```python
from build123d import *

# Parameters (mm, degrees)
BOSS_EXTRUDE1_DEPTH = 15.6
BOSS_EXTRUDE2_DEPTH = 6.75
BOSS_EXTRUDE3_DEPTH = 4
BOSS_EXTRUDE4_DEPTH = 3
SKETCH5_R           = 1.65
CUT_EXTRUDE1_DEPTH  = 8
SKETCH6_R           = 1.65
CUT_EXTRUDE2_DEPTH  = 27.35
CUT_EXTRUDE3_START  = -3
CUT_EXTRUDE3_DEPTH  = 2.6
CUT_EXTRUDE4_DEPTH  = 20
SKETCH9_W           = 15.8100889
SKETCH9_H           = 107.753083684
SKETCH9_W_2         = 8.2399111
SKETCH9_H_2         = 107.633309651
CUT_EXTRUDE5_DEPTH  = 10
SKETCH10_R          = 0.625
CUT_EXTRUDE6_DEPTH  = 30


with BuildPart() as part:
    # Sketch1 → Boss-Extrude1 (new body)
    with BuildSketch(Plane.XY):
        Polygon((-11.65, 6.6), (11.35, 6.6), (11.35, -6.2), (23.85, -6.2), (23.85, 8.35), (-24.15, 8.35), (-24.15, -6.2), (-11.65, -6.2), align=None)
    extrude(amount=-BOSS_EXTRUDE1_DEPTH)

    # Sketch2 → Boss-Extrude2 (add)
    with BuildSketch(Plane(origin=(0, 0, -15.6), x_dir=(-1, 0, 0), z_dir=(0, 0, -1))):
        Polygon((-16.2399111, -6.2), (-23.85, -6.2), (-23.85, 8.35), (24.2, 8.35), (24.2, -6.2), (16.0600889, -6.2), (16.0600889, 6.6), (-16.2399111, 6.6), align=None)
    extrude(amount=BOSS_EXTRUDE2_DEPTH)

    # Sketch3 → Boss-Extrude3 (add)
    with BuildSketch(Plane.XY):
        with BuildLine():
            Line((-24.15, 8.35), (23.85, 8.35))
            Line((23.85, 8.35), (23.85, 1.000334142))
            Line((23.85, 1.000334142), (23.85, -108.560334142))
            ThreePointArc((23.85, -108.560334142), (0.155860803, -114.961112509), (-24.15, -111.554159822))
            Line((-24.15, -111.554159822), (-24.15, 3.741161814))
            Line((-24.15, 3.741161814), (-24.15, 8.35))
        make_face()
    extrude(amount=BOSS_EXTRUDE3_DEPTH)

    # Sketch4 → Boss-Extrude4 (add)
    with BuildSketch(Plane(origin=(0, 0, 0), x_dir=(-1, 0, 0), z_dir=(0, 0, -1))):
        with BuildLine():
            ThreePointArc((10.093422233, -114.741481463), (13.037755905, -114.358456249), (15.9600889, -113.833309651))
            Line((15.9600889, -113.833309651), (15.9600889, -35.2))
            Line((15.9600889, -35.2), (10.093422233, -35.2))
            Line((10.093422233, -35.2), (10.093422233, -114.741481463))
        make_face()
        with BuildLine():
            ThreePointArc((1.026755567, -115.023412344), (3.960432973, -115.079264216), (6.893422233, -114.994667814))
            Line((6.893422233, -114.994667814), (6.893422233, -35.2))
            Line((6.893422233, -35.2), (1.026755567, -35.2))
            Line((1.026755567, -35.2), (1.026755567, -115.023412344))
        make_face()
        with BuildLine():
            ThreePointArc((-8.0399111, -113.953083684), (-5.116842896, -114.448405849), (-2.173244433, -114.801817592))
            Line((-2.173244433, -114.801817592), (-2.173244433, -35.2))
            Line((-2.173244433, -35.2), (-8.0399111, -35.2))
            Line((-8.0399111, -35.2), (-8.0399111, -113.953083684))
        make_face()
    extrude(amount=BOSS_EXTRUDE4_DEPTH)

    # Sketch5 → Cut-Extrude1 (cut, through all)
    with BuildSketch(Plane(origin=(0, 0, -3), x_dir=(-1, 0, 0), z_dir=(0, 0, -1))):
        with Locations((3.9600889, -46.2)):
            Circle(SKETCH5_R)
        with Locations((12.4600889, -46.2)):
            Circle(SKETCH5_R)
        with Locations((-4.5399111, -46.2)):
            Circle(SKETCH5_R)
        with Locations((12.4600889, -105.2)):
            Circle(SKETCH5_R)
        with Locations((-4.5399111, -105.2)):
            Circle(SKETCH5_R)
    extrude(amount=-CUT_EXTRUDE1_DEPTH, mode=Mode.SUBTRACT)

    # Sketch6 → Cut-Extrude2 (cut, through all)
    with BuildSketch(Plane(origin=(0, 0, -22.35), x_dir=(-1, 0, 0), z_dir=(0, 0, -1))):
        with Locations((-20.1399111, -2.18)):
            Circle(SKETCH6_R)
        with Locations((-20.1399111, 3.82)):
            Circle(SKETCH6_R)
        with Locations((19.9600889, -2.18)):
            Circle(SKETCH6_R)
        with Locations((19.9600889, 3.82)):
            Circle(SKETCH6_R)
    extrude(amount=-CUT_EXTRUDE2_DEPTH, mode=Mode.SUBTRACT)

    # Sketch7 → Cut-Extrude3 (cut)
    with BuildSketch(Plane(origin=(0, 0, -22.35), x_dir=(-1, 0, 0), z_dir=(0, 0, -1)).offset(CUT_EXTRUDE3_START)):
        Polygon((18.314640633, 0.67), (16.669192365, -2.18), (18.314640633, -5.03), (21.605537167, -5.03), (23.250985434, -2.18), (21.605537167, 0.67), align=None)
        Polygon((21.605537167, 6.67), (18.314640633, 6.67), (16.669192365, 3.82), (18.314640633, 0.97), (21.605537167, 0.97), (23.250985434, 3.82), align=None)
        Polygon((-21.785359367, 6.67), (-23.430807635, 3.82), (-21.785359367, 0.97), (-18.494462833, 0.97), (-16.849014566, 3.82), (-18.494462833, 6.67), align=None)
        Polygon((-21.785359367, 0.67), (-23.430807635, -2.18), (-21.785359367, -5.03), (-18.494462833, -5.03), (-16.849014566, -2.18), (-18.494462833, 0.67), align=None)
    extrude(amount=-CUT_EXTRUDE3_DEPTH, mode=Mode.SUBTRACT)

    # Sketch8 → Cut-Extrude4 (cut)
    with BuildSketch(Plane.ZY.offset(-11.35)):
        Polygon((0, 6.6), (-4.810139763, 6.6), (-8, 1.075), (-4.810139763, -4.45), (0, -4.45), align=None)
    extrude(amount=-CUT_EXTRUDE4_DEPTH, mode=Mode.SUBTRACT)

    # Sketch9 → Cut-Extrude5 (cut)
    with BuildSketch(Plane(origin=(0, 0, 0), x_dir=(-1, 0, 0), z_dir=(0, 0, -1))):
        with Locations((-15.94495555, -60.076541842)):
            Rectangle(SKETCH9_W, SKETCH9_H)
        with Locations((20.08004445, -60.016654826)):
            Rectangle(SKETCH9_W_2, SKETCH9_H_2)
    extrude(amount=-CUT_EXTRUDE5_DEPTH, mode=Mode.SUBTRACT)

    # Sketch10 → Cut-Extrude6 (cut)
    with BuildSketch(Plane(origin=(0, 0, -15.6), x_dir=(-1, 0, 0), z_dir=(0, 0, -1))):
        with Locations((13.8100889, 0.32)):
            Circle(SKETCH10_R)
        with Locations((-13.9899111, 0.32)):
            Circle(SKETCH10_R)
    extrude(amount=-CUT_EXTRUDE6_DEPTH, mode=Mode.SUBTRACT)


solid = part.part
```
Geometry: final body of the model. Coordinates: model frame, mm. A direction names the side the tool comes from. Coordinates: 2 decimals unless noted, no trailing zeros. Order: outer loops, then holes, each group sorted by start corner. A loop starts at its lowest first (then second) coordinate and runs counter-clockwise, first axis right, second up.
Item 1: Section query C-C (y = -46.2). Output: boundary loops of the cut face in (x, z).
Answer:
outline: (-15.96, -3) - (-14.11, -3) - (-14.11, 4) - (-15.96, 4) - close; (-10.81, -3) - (-10.09, -3) - (-10.09, 0) - (-6.89, 0) - (-6.89, -3) - (-5.61, -3) - (-5.61, 4) - (-10.81, 4) - close; (-2.31, -3) - (-1.03, -3) - (-1.03, 0) - (2.17, 0) - (2.17, -3) - (2.89, -3) - (2.89, 4) - (-2.31, 4) - close; (6.19, -3) - (8.04, -3) - (8.04, 4) - (6.19, 4) - close
Item 2: Contact query for flat-ended pins moving along their axis: P1, Ø3.5, axis at y = -58, z = -1, coming from the -X side; P2, Ø2, axis at x = 20, z = -17.5, coming from the -Y side; P3, Ø1, axis at x = -8.5, y = -88, coming from the -Z side. Output: stop coordinate, or through.
Answer:
P1: stops at x = -15.96
P2: stops at y = -6.2
P3: stops at z = 0
Item 3: Section query A-A (y = -105.2). Output: boundary loops of the cut face in (x, z), then the cut area to 3 significant figures.
Answer:
outline: (-15.96, -3) - (-14.11, -3) - (-14.11, 4) - (-15.96, 4) - close; (-10.81, -3) - (-10.09, -3) - (-10.09, 0) - (-6.89, 0) - (-6.89, -3) - (-1.03, -3) - (-1.03, 0) - (2.17, 0) - (2.17, -3) - (2.89, -3) - (2.89, 4) - (-10.81, 4) - close; (6.19, -3) - (8.04, -3) - (8.04, 4) - (6.19, 4) - close
area: 103 mm2
Item 4: Section query D-D (y = -75). Output: boundary loops of the cut face in (x, z), then the cut area to 3 significant figures.
Answer:
outline: (-15.96, -3) - (-10.09, -3) - (-10.09, 0) - (-6.89, 0) - (-6.89, -3) - (-1.03, -3) - (-1.03, 0) - (2.17, 0) - (2.17, -3) - (8.04, -3) - (8.04, 4) - (-15.96, 4) - close
area: 149 mm2
Item 5: Access query for faces 4 (the face through (-5, -53, 4)), 5 (the face through (20.5, -3.79, -11.03)), 6 (the face through (18.7, -0.9, -19.35)), 7 (the face through (-4, -75, -3)), 8 (the face through (18, -4.45, -2)). Directions: +Z, -Z, +X, -X, +Y, -Y. A direction counts if a zero-diameter tool reaches every point of the face in a straight line with its end or side. Return the directions, or none.
Answer:
face 4: +Z, +X, -X, +Y, -Y
face 5: +Z, -Z
face 6: none
face 7: -Z, +X, -X, -Y
face 8: +X
Item 6: Material intervals for line 1 along X through (y, z) = (-63.5, -2.75); line 2 along Y through (x, z) = (-18.5, 1); line 3 along X through (y, z) = (-0.5, -18.5), sorted ascending.
Answer:
line 1: x = -15.96 to -10.09, -6.89 to -1.03, 2.17 to 8.04
line 2: y = -6.2 to -2.95, -1.41 to 3.05, 4.59 to 8.35
line 3: x = -24.2 to -22.28, -17.64 to -16.06, 16.24 to 17.82, 22.46 to 23.85
Item 7: Section query B-B (z = 2). State how many separate pieces and enclosed holes the cut face has, then the cut area to 3 significant figures.
Answer:
separate pieces: 1
enclosed holes: 11
area: 3,220 mm2
Item 8: Draft query along X for faces 1 (the face through (-15.96, -61, 0)), 2 (the face through (5, -35.2, -1)), 3 (the face through (-15, 0, -15.6)). Return one class per face: released by +X, released by -X, zero draft, split by the parting line, or undercut.
Answer:
face 1: released by -X
face 2: zero draft
face 3: undercut
